Here's how the part is built. I have some questions about the finished solid (model axes, mm). Face numbers are marked on the shaded views. A direction names the side the tool comes from. Give positions to 0.01 mm unless a question says otherwise; leave off trailing zeros. Write each loop counter-clockwise with the first axis right and the second up, starting at its lowest first coordinate (ties: lowest second). Pieces come first, ordered by that corner, then holes. Notation, with made-up numbers: (-1, -13.5) - (42, -13.5) arc R19 ccw to (42, 8.5) - close; hole circle Ø11 at (87, 43). An arc over 180 degrees is marked (long way). Use one line per item in the form item = value. Start each with the question number.
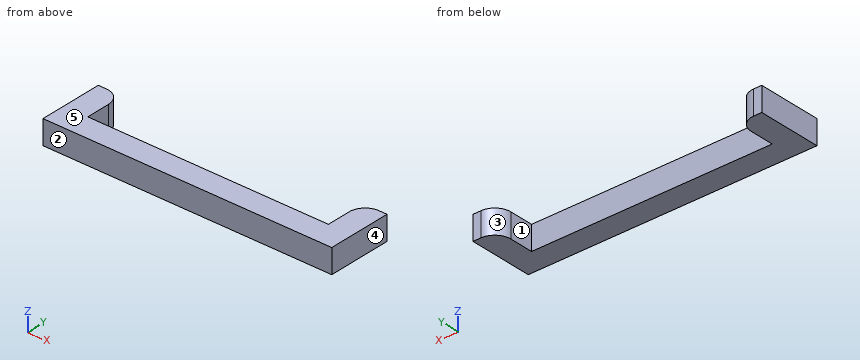
from build123d import *

# Parameters (mm, degrees)
F0_W     = 30
F0_H     = 3
F1_DEPTH = 3


with BuildPart() as f1:
    # F0 (on Top) → F1 (new body)
    with BuildSketch(Plane.XY):
        with Locations((-4.936537, 0.902144)):
            Rectangle(F0_W, F0_H)
        with BuildLine():
            Line((10.063463, 2.402144), (10.063463, -0.597856))
            Line((10.063463, -0.597856), (13.063463, -0.597856))
            Line((13.063463, -0.597856), (13.063463, 7.402144))
            Line((13.063463, 7.402144), (12.063463, 7.402144))
            ThreePointArc((12.063463, 7.402144), (10.649249, 6.816358), (10.063463, 5.402144))
            Line((10.063463, 5.402144), (10.063463, 2.402144))
        make_face()
        with BuildLine():
            Line((-22.936537, -0.597856), (-19.936537, -0.597856))
            Line((-19.936537, -0.597856), (-19.936537, 2.402144))
            Line((-19.936537, 2.402144), (-19.936537, 5.402144))
            ThreePointArc((-19.936537, 5.402144), (-20.522324, 6.816358), (-21.936537, 7.402144))
            Line((-21.936537, 7.402144), (-22.936537, 7.402144))
            Line((-22.936537, 7.402144), (-22.936537, -0.597856))
        make_face()
    extrude(amount=F1_DEPTH)


solid = f1.part
1. For the marked faces 1 and 2, which set-ups out of +Z, -Z, +X, -X, +Y, -Y let a thin tool reach every point of the face, with its end or its side?
2. We'd pull the mould along X, two halves only. Please class the marked faces 3, 4 and 5: pulls with the +X half, pulls with the -X half, needs draft (parallel to the pull), parting line crosses it, or undercut.
3. Please list where these lines run through material, in increasing order: line 1 (X direction, y = 2.75, z = 2.4); line 2 (Y direction, x = 2, z = 2.5); line 3 (X direction, y = 6.5, z = 1.05).
4. I want a section at C-C, the plane x = 11. List the corners of the cut face in (y, z) for me, then the cut area to 3 significant figures.
5. I want a section at B-B, the plane x = 3.5. List the corners of the cut face in (y, z) for me.
6. I want a section at A-A, the plane z = 0.4. List the corners of the cut face in (x, y) for me.
7. For P1, Ø1, axis at x = 4, z = 2.5, coming from the +Y side, with a flat end and sliding along its axis, tell me the tip position at first contact or that it passes through.
Result sheet:
q1.face_1 = +Z, -Z, +Y
q1.face_2 = +Z, -Z, +X, -X, -Y
q2.face_3 = undercut
q2.face_4 = pulls with the +X half
q2.face_5 = needs draft
q3.line_1 = -22.94 to -19.94, 10.06 to 13.06
q3.line_2 = -0.6 to 2.4
q3.line_3 = -22.94 to -20.26, 10.39 to 13.06
q4.outline = (-0.6, 0) - (7.1, 0) - (7.1, 3) - (-0.6, 3) - close
q4.area = 23.1 mm2
q5.outline = (-0.6, 0) - (2.4, 0) - (2.4, 3) - (-0.6, 3) - close
q6.outline = (-22.94, -0.6) - (13.06, -0.6) - (13.06, 7.4) - (12.06, 7.4) arc R2 ccw to (10.06, 5.4) - (10.06, 2.4) - (-19.94, 2.4) - (-19.94, 5.4) arc R2 ccw to (-21.94, 7.4) - (-22.94, 7.4) - close
q7.P1 = 2.4
